For this review, take the finished solid that the model builds, in its own axes (mm). Face numbers are marked on the shaded views. A direction names the side the tool comes from. Coordinates: 2 decimals unless noted, no trailing zeros. Write each loop counter-clockwise with the first axis right and the second up, starting at its lowest first coordinate (ties: lowest second). Pieces come first, ordered by that corner, then holes. Notation, with made-up numbers: M 42,26 L 70,26 A30 ccw 70,49 Z; hole C 84.5,23.25 d11. An arc over 180 degrees is marked long. One line per question, with ' | ' between items.
Autodesk Fusion 360 part; units mm, degrees
ref_plane "工作平面1" through (0, 0, 0) normal (0, 0, 1) x (1, 0, 0)
sketch "草图1" plane through (0, 0, 0) normal (0, 0, 1) x (1, 0, 0)
  line L0 (-25, -9) -> (25, -9)
  line L1 (25, -9) -> (25, 9)
  line L2 (25, 9) -> (-25, 9)
  line L3 (-25, 9) -> (-25, -9)
extrude "Coupon base" add sketch "草图1" along normal blind 2
ref_plane "工作平面2" through (0, 0, 2) normal (0, 0, 1) x (1, 0, 0)
sketch "草图2" plane through (0, 0, 2) normal (0, 0, 1) x (1, 0, 0)
  line L0 (-25, -9) -> (-20.59, -9)
  line L1 (-20.59, -9) -> (-20.59, 9)
  line L2 (-20.59, 9) -> (-25, 9)
  line L3 (-25, 9) -> (-25, -9)
ref_plane "工作平面3" through (0, 0, 7.2) normal (0, 0, 1) x (1, 0, 0)
sketch "草图3" plane through (0, 0, 7.2) normal (0, 0, 1) x (1, 0, 0)
  line L0 (-25, -9) -> (-16.43, -9)
  line L1 (-16.43, -9) -> (-16.43, 9)
  line L2 (-16.43, 9) -> (-25, 9)
  line L3 (-25, 9) -> (-25, -9)
loft "Coupon dovetail rail" add profiles "草图2", "草图3" section 1 section 2
ref_plane "工作平面4" through (0, 0, 2) normal (0, 0, 1) x (1, 0, 0)
sketch "草图4" plane through (0, 0, 2) normal (0, 0, 1) x (1, 0, 0)
  line L0 (20.59, -9) -> (25, -9)
  line L1 (25, -9) -> (25, 9)
  line L2 (25, 9) -> (20.59, 9)
  line L3 (20.59, 9) -> (20.59, -9)
ref_plane "工作平面5" through (0, 0, 7.2) normal (0, 0, 1) x (1, 0, 0)
sketch "草图5" plane through (0, 0, 7.2) normal (0, 0, 1) x (1, 0, 0)
  line L0 (16.43, -9) -> (25, -9)
  line L1 (25, -9) -> (25, 9)
  line L2 (25, 9) -> (16.43, 9)
  line L3 (16.43, 9) -> (16.43, -9)
loft "Coupon dovetail rail (1)" add profiles "草图4", "草图5" section 1 section 2
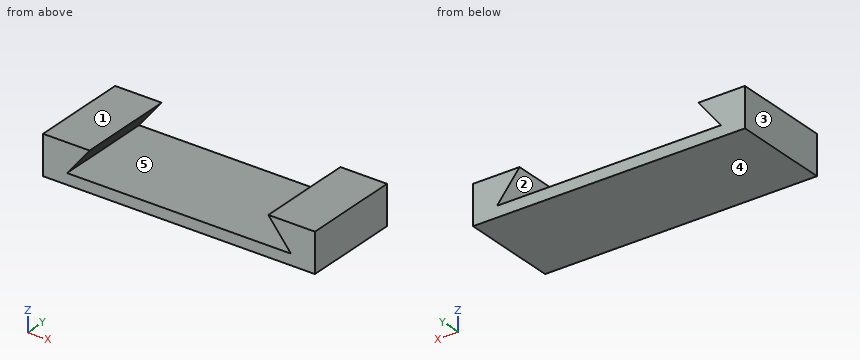
1) The part is to be moulded in two halves that separate along X. For the marked faces 1, 2 and 3, say which applies: +X half, -X half, draft (parallel to the pull), parting line (faces both ways), or undercut.
Responses:
face 1: draft | face 2: undercut | face 3: -X half
2) We need section C-C on y = -5. State the section outline as (x, z) points, then the cut area to 3 significant figures.
Responses:
outline: M -25,0 L 25,0 L 25,7.2 L 16.43,7.2 L 20.59,2 L -20.59,2 L -16.43,7.2 L -25,7.2 Z | area: 167 mm^2
3) Machinability: for the marked faces 4 and 5, which of the approach directions +Z, -Z, +X, -X, +Y, -Y give a long, thin tool a straight path to every point of the face, cutting with its end or side? Answer none if there is none.
Responses:
face 4: -Z, +X, -X, +Y, -Y | face 5: +Y, -Y
4) We need section D-D on x = -4. State the section outline as (y, z) points.
Responses:
outline: M -9,0 L 9,0 L 9,2 L -9,2 Z
5) We need section A-A on z = 2.5. State the section outline as (x, y) points.
Responses:
outline: M -25,-9 L -20.19,-9 L -20.19,9 L -25,9 Z; M 20.19,-9 L 25,-9 L 25,9 L 20.19,9 Z
6) We need section B-B on z = 5.5. State the section outline as (x, y) points, then the cut area to 3 significant figures.
Responses:
outline: M -25,-9 L -17.79,-9 L -17.79,9 L -25,9 Z; M 17.79,-9 L 25,-9 L 25,9 L 17.79,9 Z | area: 260 mm^2
7) Insertion check: pin 1 Ø5.5 at (x, y) = (-6.5, -1) entering from +Z. The pin has a flat end and moves straight along its axis. Give the tip position at first contact, or say it passes through.
Responses:
pin 1: z = 2
8) To check wall thickness, follow line 1 along Z through (x, y) = (-8.5, -0.25); line 2 along X through (y, z) = (5.75, 3.5); line 3 along X through (y, z) = (-2, 5.75). State the ranges of each line that lie inside material, in increasing order. Write a range as [from, to].
Responses:
line 1: [0, 2] | line 2: [-25, -19.39], [19.39, 25] | line 3: [-25, -17.59], [17.59, 25]
